Geometry check sheet. Reference: the model listing, model coordinates, mm. Face numbers are marked on the shaded views. A direction names the side the tool comes from. Coordinates: 2 decimals unless noted, no trailing zeros. Order: outer loops, then holes, each group sorted by start corner. A loop starts at its lowest first (then second) coordinate and runs counter-clockwise, first axis right, second up. Notation, with made-up numbers: M 53,-30.5 L 83,-30.5 A28 cw 83,-8.5 Z; hole C -4.75,30 d11. An arc over 180 degrees is marked long. One line per item, written item: value. Start each with the question number.
1) Thickness scan on L1, parallel to Z at x = 27.5, y = 41.25 (3 decimals); L2, parallel to Z at x = 16, y = 24.5; L3, parallel to Z at x = 23.5, y = 19. Record the ranges inside material, lowest first. Write a range as from..to.
2) Draft check along Y on the marked faces 1, 2 and 3. Enter one of: pulls with the +Y half, pulls with the -Y half, needs draft (parallel to the pull), parting line crosses it, or undercut.
3) Access from +Z, -Z, +X, -X, +Y, -Y to the whole of each face (thin tool, end or side, straight path). Record for the marked faces 4, 5, 6, 7 and 8.
4) Sectioned sample at A-A, the plane z = -11. Enter the section's corners in (x, y), then the cut area to 3 significant figures.
5) Sectioned sample at B-B, the plane y = 34. State how many separate pieces and enclosed holes the cut face has, then the cut area to 3 significant figures.
6) Go/stop test with flat-tipped pins: P1, Ø5.5, axis at x = 26.5, y = 5.5, coming from the +Z side; P2, Ø3, axis at x = 8, z = -2.5, coming from the +Y side; P3, Ø1, axis at y = 25.5, z = -22, coming from the +X side; P4, Ø2, axis at x = 8, y = 6.49, coming from the +Z side. Record where each tip stops, or that it passes through.
```python
from build123d import *

# Parameters (mm, degrees)
SKETCH11_W          = 35
SKETCH11_H          = 27
BOSS_EXTRUDE6_DEPTH = 10
SKETCH12_R          = 1.7
CUT_EXTRUDE3_DEPTH  = 11
SKETCH13_W          = 35
SKETCH13_H          = 8
BOSS_EXTRUDE7_DEPTH = 22
SKETCH14_W          = 35
SKETCH14_H          = 10
BOSS_EXTRUDE8_DEPTH = 35
SKETCH17_W          = 35
SKETCH17_H          = 35
CUT_EXTRUDE6_DEPTH  = 1.2
SKETCH18_W          = 1.1
SKETCH18_H          = 35
CUT_EXTRUDE7_DEPTH  = 1.2
SKETCH19_R          = 1.7
CUT_EXTRUDE8_DEPTH  = 44
CUT_EXTRUDE9_DEPTH  = 2.5
CUT_EXTRUDE10_DEPTH = 2.5
BOSS_EXTRUDE9_DEPTH = 35
SKETCH23_R          = 1.6
CUT_EXTRUDE11_DEPTH = 15
CUT_EXTRUDE12_DEPTH = 2
CUT_EXTRUDE13_DEPTH = 2


with BuildPart() as part:
    # Sketch11 → Boss-Extrude6 (new body)
    with BuildSketch(Plane(origin=(0, 0, 12.5), x_dir=(1, 0, 0), z_dir=(0, -1, 0))):
        with Locations((17.5, -13.5)):
            Rectangle(SKETCH11_W, SKETCH11_H)
    extrude(amount=BOSS_EXTRUDE6_DEPTH)

    # Sketch12 → Cut-Extrude3 (cut, through all)
    with BuildSketch(Plane.XZ.offset(10)):
        with Locations((10, 9)):
            Circle(SKETCH12_R)
        with Locations((25, 9)):
            Circle(SKETCH12_R)
        with Locations((25, -11)):
            Circle(SKETCH12_R)
        with Locations((10, -11)):
            Circle(SKETCH12_R)
    extrude(amount=-CUT_EXTRUDE3_DEPTH, mode=Mode.SUBTRACT)

    # Sketch13 → Boss-Extrude7 (add)
    with BuildSketch(Plane.XZ.offset(10)):
        with Locations((17.5, -18.5)):
            Rectangle(SKETCH13_W, SKETCH13_H)
        with Locations((17.5, 16.5)):
            Rectangle(SKETCH13_W, SKETCH13_H)
    extrude(amount=-BOSS_EXTRUDE7_DEPTH)

    # Sketch14 → Boss-Extrude8 (add)
    with BuildSketch(Plane(origin=(0, 12, 0), x_dir=(1, 0, 0), z_dir=(0, 1, 0))):
        with Locations((17.5, -15.5)):
            Rectangle(SKETCH14_W, SKETCH14_H)
        with Locations((17.5, 17.5)):
            Rectangle(SKETCH14_W, SKETCH14_H)
    extrude(amount=BOSS_EXTRUDE8_DEPTH)

    # Sketch17 → Cut-Extrude6 (cut)
    with BuildSketch(Plane.XY.offset(20.5)):
        with Locations((17.5, 29.5)):
            Rectangle(SKETCH17_W, SKETCH17_H)
    extrude(amount=-CUT_EXTRUDE6_DEPTH, mode=Mode.SUBTRACT)

    # Sketch18 → Cut-Extrude7 (cut)
    with BuildSketch(Plane(origin=(0, 0, -22.5), x_dir=(-1, 0, 0), z_dir=(0, 0, -1))):
        with Locations((-32.45, 29.5)):
            Rectangle(SKETCH18_W, SKETCH18_H)
        with Locations((-34.45, 29.5)):
            Rectangle(SKETCH18_W, SKETCH18_H)
        with Locations((-30.45, 29.5)):
            Rectangle(SKETCH18_W, SKETCH18_H)
        with Locations((-28.45, 29.5)):
            Rectangle(SKETCH18_W, SKETCH18_H)
        with Locations((-26.45, 29.5)):
            Rectangle(SKETCH18_W, SKETCH18_H)
        with Locations((-24.45, 29.5)):
            Rectangle(SKETCH18_W, SKETCH18_H)
        with Locations((-22.45, 29.5)):
            Rectangle(SKETCH18_W, SKETCH18_H)
        with Locations((-20.45, 29.5)):
            Rectangle(SKETCH18_W, SKETCH18_H)
        with Locations((-18.45, 29.5)):
            Rectangle(SKETCH18_W, SKETCH18_H)
        with Locations((-16.45, 29.5)):
            Rectangle(SKETCH18_W, SKETCH18_H)
        with Locations((-14.45, 29.5)):
            Rectangle(SKETCH18_W, SKETCH18_H)
        with Locations((-12.45, 29.5)):
            Rectangle(SKETCH18_W, SKETCH18_H)
        with Locations((-10.45, 29.5)):
            Rectangle(SKETCH18_W, SKETCH18_H)
        with Locations((-8.45, 29.5)):
            Rectangle(SKETCH18_W, SKETCH18_H)
        with Locations((-6.45, 29.5)):
            Rectangle(SKETCH18_W, SKETCH18_H)
        with Locations((-4.45, 29.5)):
            Rectangle(SKETCH18_W, SKETCH18_H)
        with Locations((-2.45, 29.5)):
            Rectangle(SKETCH18_W, SKETCH18_H)
        with Locations((-0.45, 29.5)):
            Rectangle(SKETCH18_W, SKETCH18_H)
    extrude(amount=-CUT_EXTRUDE7_DEPTH, mode=Mode.SUBTRACT)

    # Sketch19 → Cut-Extrude8 (cut, through all)
    with BuildSketch(Plane(origin=(0, 0, -22.5), x_dir=(-1, 0, 0), z_dir=(0, 0, -1))):
        with Locations((-27, 6.485099569)):
            Circle(SKETCH19_R)
        with Locations((-8, 6.485099569)):
            Circle(SKETCH19_R)
        with Locations((-17.5, 43)):
            Circle(SKETCH19_R)
    extrude(amount=-CUT_EXTRUDE8_DEPTH, mode=Mode.SUBTRACT)

    # Sketch20 → Cut-Extrude9 (cut)
    with BuildSketch(Plane.XY.offset(-14.5)):
        Polygon((28.5, 3.887023357), (30, 6.485099569), (28.5, 9.08317578), (25.5, 9.08317578), (24, 6.485099569), (25.5, 3.887023357), align=None)
        Polygon((9.5, 3.887023357), (11, 6.485099569), (9.5, 9.08317578), (6.5, 9.08317578), (5, 6.485099569), (6.5, 3.887023357), align=None)
    extrude(amount=-CUT_EXTRUDE9_DEPTH, mode=Mode.SUBTRACT)

    # Sketch21 → Cut-Extrude10 (cut)
    with BuildSketch(Plane(origin=(0, 0, 12.5), x_dir=(-1, 0, 0), z_dir=(0, 0, -1))):
        Polygon((-6.45, 3.800420817), (-4.9, 6.485099569), (-6.45, 9.16977832), (-9.55, 9.16977832), (-11.1, 6.485099569), (-9.55, 3.800420817), align=None)
        Polygon((-25.45, 3.800420817), (-23.9, 6.485099569), (-25.45, 9.16977832), (-28.55, 9.16977832), (-30.1, 6.485099569), (-28.55, 3.800420817), align=None)
    extrude(amount=-CUT_EXTRUDE10_DEPTH, mode=Mode.SUBTRACT)

    # Sketch22 → Boss-Extrude9 (add)
    with BuildSketch(Plane(origin=(0, 47, 0), x_dir=(1, 0, 0), z_dir=(0, 1, 0))):
        with BuildLine():
            Line((35, 21.3), (35, 12.5))
            ThreePointArc((35, 12.5), (39.4, 16.9), (35, 21.3))
        make_face()
        with BuildLine():
            Line((35, -10.5), (35, -19.3))
            ThreePointArc((35, -19.3), (39.4, -14.9), (35, -10.5))
        make_face()
        with BuildLine():
            Line((0, 21.3), (0, 12.5))
            ThreePointArc((0, 12.5), (-4.4, 16.9), (0, 21.3))
        make_face()
        with BuildLine():
            Line((0, -10.5), (0, -19.3))
            ThreePointArc((0, -19.3), (-4.4, -14.9), (0, -10.5))
        make_face()
    extrude(amount=-BOSS_EXTRUDE9_DEPTH)

    # Sketch23 → Cut-Extrude11 (cut)
    with BuildSketch(Plane(origin=(0, 47, 0), x_dir=(1, 0, 0), z_dir=(0, 1, 0))):
        with Locations((7.5, 17.352667036)):
            Circle(SKETCH23_R)
        with Locations((27.5, 16.995008076)):
            Circle(SKETCH23_R)
        with Locations((27.5, -14.559659808)):
            Circle(SKETCH23_R)
        with Locations((7.5, -14.559659808)):
            Circle(SKETCH23_R)
    extrude(amount=-CUT_EXTRUDE11_DEPTH, mode=Mode.SUBTRACT)

    # Sketch24 → Cut-Extrude12 (cut)
    with BuildSketch(Plane(origin=(0, 0, 10.5), x_dir=(-1, 0, 0), z_dir=(0, 0, -1))):
        Polygon((-15.95, 40.315321248), (-14.4, 43), (-15.95, 45.684678752), (-19.05, 45.684678752), (-20.6, 43), (-19.05, 40.315321248), align=None)
    extrude(amount=-CUT_EXTRUDE12_DEPTH, mode=Mode.SUBTRACT)

    # Sketch25 → Cut-Extrude13 (cut)
    with BuildSketch(Plane.XY.offset(-12.5)):
        Polygon((19.05, 40.315321248), (20.6, 43), (19.05, 45.684678752), (15.95, 45.684678752), (14.4, 43), (15.95, 40.315321248), align=None)
    extrude(amount=-CUT_EXTRUDE13_DEPTH, mode=Mode.SUBTRACT)


solid = part.part
```
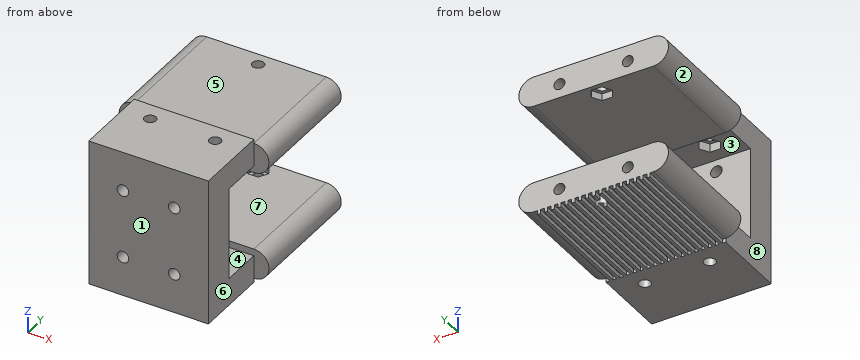
Final values:
1. L1: z = -22.5..-18.595, -15.395..-12.5, 10.5..12.96, 16.16..19.3
1. L2: z = -21.3..-12.5, 10.5..19.3
1. L3: z = -22.5..-12.5, 10.5..19.3
2. face 1: pulls with the -Y half
2. face 2: needs draft
2. face 3: undercut
3. face 4: +X, -X
3. face 5: +Z, +X, -X, +Y
3. face 6: +Z, -Z, +X, -Y
3. face 7: +X, -X, +Y
3. face 8: +Z, -Z, -X, -Y
4. outline: M 0,-10 L 8.3,-10 L 8.3,0 L 0,0 Z; M 11.7,-10 L 23.3,-10 L 23.3,0 L 11.7,0 Z; M 26.7,-10 L 35,-10 L 35,0 L 26.7,0 Z
4. area: 282 mm^2
5. separate pieces: 2
5. enclosed holes: 4
5. area: 724 mm^2
6. P1: stops at z = 20.5
6. P2: stops at y = 0
6. P3: stops at x = 33.9
6. P4: passes through
